```python
from build123d import *

# Parameters (mm, degrees)
BOSS_EXTRUDE5_DEPTH = 355
SKETCH7_W           = 2
SKETCH7_H           = 27.946586717
CUT_EXTRUDE1_DEPTH  = 33
SKETCH9_W           = 2
SKETCH9_H           = 28
CUT_EXTRUDE2_DEPTH  = 33
FILLET4_R           = 1
FILLET5_R           = 1
FILLET6_R           = 1
FILLET7_R           = 1


with BuildPart() as part:
    # Sketch6 → Boss-Extrude5 (new body)
    with BuildSketch(Plane(origin=(0, 0, 0), x_dir=(0, 0, -1), z_dir=(1, 0, 0))):
        Polygon((0, 3), (0, 0), (31, 0), (31, 26), (26, 26), (26, 31), (18, 31), (18, 33), (28, 33), (28, 28), (33, 28), (33, -2), (-2, -2), (-2, 3), align=None)
    extrude(amount=-BOSS_EXTRUDE5_DEPTH)

    # Sketch7 → Cut-Extrude1 (cut)
    with BuildSketch(Plane.XY.offset(2)):
        with Locations((-1, 11.973293359)):
            Rectangle(SKETCH7_W, SKETCH7_H)
    extrude(amount=-CUT_EXTRUDE1_DEPTH, mode=Mode.SUBTRACT)

    # Sketch9 → Cut-Extrude2 (cut)
    with BuildSketch(Plane.XY.offset(2)):
        with Locations((-354, 12)):
            Rectangle(SKETCH9_W, SKETCH9_H)
    extrude(amount=-CUT_EXTRUDE2_DEPTH, mode=Mode.SUBTRACT)

    # Fillet4
    fillet4_edges = [part.edges().sort_by_distance(p)[0] for p in [
        (-177.5, 26, -31),
        (-177.5, 31, -26),
        (-177.5, 33, -28),
        (-177.5, 28, -28),
        (-177.5, 28, -33),
    ]]
    fillet(fillet4_edges, radius=FILLET4_R)

    # Fillet5
    fillet5_edges = [part.edges().sort_by_distance(p)[0] for p in [
        (-177.5, -2, -33),
    ]]
    fillet(fillet5_edges, radius=FILLET5_R)

    # Fillet6
    fillet6_edges = [part.edges().sort_by_distance(p)[0] for p in [
        (-177.5, 0, -31),
    ]]
    fillet(fillet6_edges, radius=FILLET6_R)

    # Fillet7
    fillet7_edges = [part.edges().sort_by_distance(p)[0] for p in [
        (-177.5, 26, -26),
    ]]
    fillet(fillet7_edges, radius=FILLET7_R)


solid = part.part
```
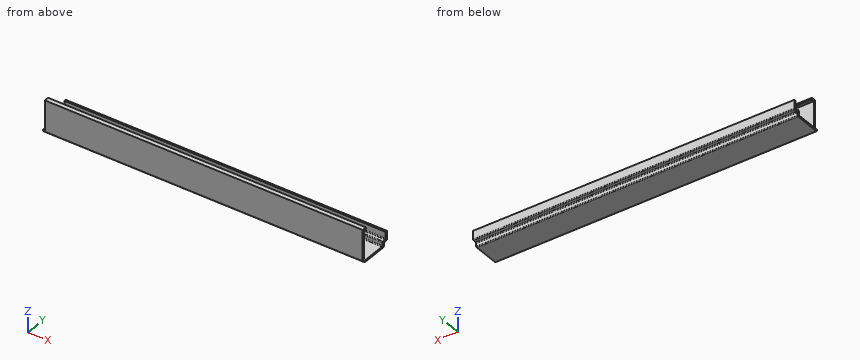
CAD build for the part. Positions are in the model's coordinates, mm. Round coordinates to 2 decimals unless told otherwise and drop trailing zeros. Write each loop counter-clockwise with the first axis right and the second up, starting at its lowest first coordinate (ties: lowest second). Pieces come first, ordered by that corner, then holes.
Item 1: Band-saw the part on A-A on z = -21.5. Write the cut outline in (x, y), then the cut area to 3 significant figures.
Filled in:
outline: (-355, 31) - (0, 31) - (0, 33) - (-355, 33) - close; (-353, -2) - (-2, -2) - (-2, 0) - (-353, 0) - close
area: 1,410 mm2
Item 2: Band-saw the part on B-B on x = -63. Write the cut outline in (y, z).
Filled in:
outline: (-2, -32) arc R1 ccw to (-1, -33) - (27, -33) arc R1 ccw to (28, -32) - (28, -29) arc R1 cw to (29, -28) - (32, -28) arc R1 ccw to (33, -27) - (33, -18) - (31, -18) - (31, -25) arc R1 cw to (30, -26) - (27, -26) arc R1 ccw to (26, -27) - (26, -30) arc R1 cw to (25, -31) - (1, -31) arc R1 cw to (0, -30) - (0, 0) - (3, 0) - (3, 2) - (-2, 2) - close
Item 3: Drill centre lines: L1, parallel to Y at x = -107.5, z = -20; L2, parallel to Y at x = -74.5, z = -29; L3, parallel to Y at x = -167, z = -1. Where is each one in solid material? Low to high.
Filled in:
L1: y = -2 to 0, 31 to 33
L2: y = -2 to 0, 26 to 28
L3: y = -2 to 0
Item 4: Drop flat-ended pins along their axis: pin 1 Ø2.5 at (x, y) = (-208.5, 31) entering from -Z; pin 2 Ø1.6 at (x, z) = (-95.5, 1) entering from +Y; pin 3 Ø2.5 at (y, z) = (1.5, -12) entering from +X; pin 4 Ø2.5 at (y, z) = (0.5, -11) entering from -X. Give the stop position or say it passes through.
Filled in:
pin 1: stops at z = -28
pin 2: stops at y = 3
pin 3: passes through
pin 4: stops at x = -353
Item 5: Band-saw the part on C-C on y = 7. Write the cut outline in (x, z), then the cut area to 3 significant figures.
Filled in:
outline: (-355, -33) - (0, -33) - (0, -31) - (-355, -31) - close
area: 710 mm2
